For this review, take the finished solid that the model builds, in its own axes (mm). A direction names the side the tool comes from. Give positions to 0.01 mm unless a question says otherwise; leave off trailing zeros. Order: outer loops, then holes, each group sorted by start corner. A loop starts at its lowest first (then second) coordinate and runs counter-clockwise, first axis right, second up.
Item 1: Consider section C-C (x = -60). Give the boundary of the cut face in (y, z).
Item 2: Consider section B-B (y = 50). Give the boundary of the cut face in (x, z).
Item 3: For P1, Ø10, axis at y = 128.5, z = 19.5, coming from the +X side; P2, Ø12, axis at x = -24, z = 45, coming from the -Y side; P3, Ø8, axis at y = 199.5, z = 64.5, coming from the +X side, all flat-tipped, find the tip position at first contact; note any pin that passes through.
Item 4: Consider section D-D (y = 95.5). Give the boundary of the cut face in (x, z), plus the area to 3 significant figures.
Item 5: Consider section A-A (z = 51). Give the boundary of the cut face in (x, y), plus the area to 3 significant figures.
Item 6: For probe 1 along X at (y, z) = (84, 18.5); probe 2 along Z at (x, y) = (-28, 50.5) (1 decimal); probe 3 along Z at (x, y) = (-61.5, 242), list the stretches that pass through material, from the lowest coordinate up.
Item 7: The part is to be moulded in two halves that separate along X. For faces 1 (the cylindrical face through (-75, 324, 30)), 2 (the flat face through (-90, 72.9, 39.6)), 3 (the cylindrical face through (-104.78, 91.98, 18.32)), say which applies: released by +X, released by -X, zero draft, split by the parting line, or undercut.
Item 8: Machinability: for faces 4 (the flat face through (-30, 27.1, 39.6)), 5 (the flat face through (-38.6, 226.3, 71.2)), 6 (the flat face through (-59, 158, 80)), which of the approach directions +Z, -Z, +X, -X, +Y, -Y give a long, thin tool a straight path to every point of the face, cutting with its end or side? Answer none if there is none.
```python
from build123d import *

# Parameters (mm, degrees)
SKETCH1_W           = 120
SKETCH1_H           = 250
BOSS_EXTRUDE1_DEPTH = 100
CUT_EXTRUDE1_DEPTH  = 295.78805946
SKETCH3_R           = 25
CUT_EXTRUDE2_DEPTH  = 295.78805946
CUT_EXTRUDE3_DEPTH  = 60
SKETCH4_3_R         = 25
BOSS_EXTRUDE2_DEPTH = 150.7
FILLET2_R           = 12


with BuildPart() as part:
    # Sketch1 → Boss-Extrude1 (new body)
    with BuildSketch(Plane.XY):
        with Locations((-60, 125)):
            Rectangle(SKETCH1_W, SKETCH1_H)
    extrude(amount=BOSS_EXTRUDE1_DEPTH)

    # Sketch2 → Cut-Extrude1 (cut, through all)
    with BuildSketch(Plane.XY.offset(100)):
        with BuildLine():
            Line((-90, 179.498344353), (-90, 250))
            Line((-90, 250), (-120, 250))
            Line((-120, 250), (-120, 104))
            ThreePointArc((-120, 104), (-115.759222637, 126.156468376), (-103.636363636, 145.180915101))
            ThreePointArc((-103.636363636, 145.180915101), (-93.533981136, 161.034620706), (-90, 179.498344353))
        make_face()
        with BuildLine():
            Line((0, 250), (-30, 250))
            Line((-30, 250), (-30, 179.498344353))
            ThreePointArc((-30, 179.498344353), (-26.466018864, 161.034620706), (-16.363636364, 145.180915101))
            ThreePointArc((-16.363636364, 145.180915101), (-4.240777331, 126.156468297), (0, 103.999999829))
            Line((0, 103.999999829), (0, 250))
        make_face()
        with BuildLine():
            Line((-90, 100), (-90, 52.038475773))
            ThreePointArc((-90, 52.038475773), (-60, 44), (-30, 52.038475773))
            Line((-30, 52.038475773), (-30, 100))
            ThreePointArc((-30, 100), (-60, 130), (-90, 100))
        make_face()
        with BuildLine():
            ThreePointArc((-30, 52.038475773), (-60, 44), (-90, 52.038475773))
            Line((-90, 52.038475773), (-90, 0))
            Line((-90, 0), (-30, 0))
            Line((-30, 0), (-30, 52.038475773))
        make_face()
    extrude(amount=-CUT_EXTRUDE1_DEPTH, mode=Mode.SUBTRACT)

    # Sketch3 → Cut-Extrude2 (cut, through all)
    # profile 1 of 2: a face of its own
    with BuildSketch(Plane(origin=(0, 0, 0), x_dir=(0, 0, -1), z_dir=(1, 0, 0))):
        Polygon((-100, 0), (0, 0), (0, 104), (0, 145.180915101), (0, 179.498344353), (0, 250), (-100, 250), (-100, 179.498344353), (-100, 145.180915101), (-100, 104), align=None)
        with BuildLine():
            Line((-80, 100.990195136), (-80, 250))
            Line((-80, 250), (-20, 250))
            Line((-20, 250), (-20, 100.990195136))
            ThreePointArc((-20, 100.990195136), (-18.273733406, 91.861485844), (-13.333333333, 83.993463424))
            ThreePointArc((-13.333333333, 83.993463424), (-50, 0), (-86.666666667, 83.993463424))
            ThreePointArc((-86.666666667, 83.993463424), (-81.726266594, 91.861485844), (-80, 100.990195136))
        make_face(mode=Mode.SUBTRACT)
    # profile 2 of 2: a face of its own
    with BuildSketch(Plane(origin=(0, 0, 0), x_dir=(0, 0, -1), z_dir=(1, 0, 0))):
        with Locations((-50, 50)):
            Circle(SKETCH3_R)
    extrude(amount=-CUT_EXTRUDE2_DEPTH, mode=Mode.SUBTRACT)


with BuildPart() as cut_extrude2_kept_piece:
    # of the separate pieces the step leaves, the one the design keeps (cut_extrude2_pieces_kept)
    add(part.part.solids().sort_by_distance((-90, 50, 25))[0])

    # Sketch4 → Cut-Extrude3 (cut)
    with BuildSketch(Plane(origin=(0, 250, 0), x_dir=(1, 0, 0), z_dir=(0, 1, 0))):
        Polygon((-30, -62.6), (-47.4, -80), (-30, -80), align=None)
        Polygon((-90, -62.6), (-90, -80), (-72.6, -80), align=None)
        Polygon((-90, -20), (-90, -37.4), (-72.6, -20), align=None)
        Polygon((-47.4, -20), (-30, -37.4), (-30, -20), align=None)
    extrude(amount=-CUT_EXTRUDE3_DEPTH, mode=Mode.SUBTRACT)

    # Sketch4_3 → Boss-Extrude2 (add)
    with BuildSketch(Plane(origin=(0, 250, 0), x_dir=(1, 0, 0), z_dir=(0, 1, 0))):
        with Locations(Location((-60, -50, 0), (0, 0, 270))):
            Circle(SKETCH4_3_R)
    extrude(amount=BOSS_EXTRUDE2_DEPTH)

    # Fillet2
    fillet2_edges = [cut_extrude2_kept_piece.edges().sort_by_distance(p)[0] for p in [
        (-38.7, 190, 28.7),
        (-81.3, 190, 28.7),
        (-81.3, 190, 71.3),
        (-38.7, 190, 71.3),
    ]]
    fillet(fillet2_edges, radius=FILLET2_R)


solid = cut_extrude2_kept_piece.part
```
Resolved:
1. outline: (130, 20) - (250, 20) - (250, 25) - (400.7, 25) - (400.7, 75) - (250, 75) - (250, 80) - (130, 80) - close
2. outline: (-120, 0) - (-90, 0) - (-90, 25) - (-120, 25) - close; (-120, 75) - (-90, 75) - (-90, 100) - (-120, 100) - close; (-30, 0) - (0, 0) - (0, 25) - (-30, 25) - close; (-30, 75) - (0, 75) - (0, 100) - (-30, 100) - close
3. P1: stops at x = -3.27
3. P2: stops at y = 0
3. P3: stops at x = -30
4. outline: (-120, 19.39) - (-90, 19.39) - (-90, 80.61) - (-120, 80.61) - close; (-30, 19.39) - (0, 19.39) - (0, 80.61) - (-30, 80.61) - close
4. area: 3,670 mm2
5. outline: (-120, 0.01) - (-90, 0.01) - (-90, 25.02) - (-120, 25.02) - close; (-120, 74.98) - (-90, 74.98) - (-90, 100) arc R30 cw to (-30, 100) - (-30, 74.98) - (0, 74.98) - (0, 104) arc R60 ccw to (-16.36, 145.18) arc R50 cw to (-30, 179.5) - (-30, 250) - (-35.02, 250) - (-35.02, 400.7) - (-84.98, 400.7) - (-84.98, 250) - (-90, 250) - (-90, 179.5) arc R50 cw to (-103.64, 145.18) arc R60 ccw to (-120, 104) - close; (-30, 0.01) - (0, 0.01) - (0, 25.02) - (-30, 25.02) - close
5. area: 20,700 mm2
6. probe 1: x = -120 to -90, -30 to 0
6. probe 2: z = 0 to 25, 75 to 100
6. probe 3: z = 20 to 80
7. face 1: split by the parting line
7. face 2: undercut
7. face 3: zero draft
8. face 4: +Z, -Z, -Y
8. face 5: +Z, +X, +Y
8. face 6: +Z, +X, -X, +Y
